Part model, mm, in its own coordinate system. A direction names the side the tool comes from. Round coordinates to 2 decimals unless told otherwise and drop trailing zeros. Order: outer loops, then holes, each group sorted by start corner. A loop starts at its lowest first (then second) coordinate and runs counter-clockwise, first axis right, second up. Notation, with made-up numbers: (66, -35) - (85, -35) arc R23 cw to (85, 0) - close; hole circle Ø11 at (74, 84.25). An arc over 180 degrees is marked (long way). Return JSON: item names as keys, results as strings. Group by question number.
Item 1: Tool access for faces 4 (the face through (-9.76, 2.57, 2.17)), 5 (the face through (0, 25, 0)): list every direction of +Z, -Z, +X, -X, +Y, -Y with a clear straight run to the whole face (end or side of a thin tool).
Item 2: Probe probe 1 along X at (y, z) = (13.5, 0); probe 2 along X at (y, z) = (3.15, 0); probe 3 along Y at (x, z) = (2, 1). List the from-to ranges inside material, lowest first.
Item 3: Saw through at B-B on y = 6.25. List the corners of the cut face in (x, z).
Item 4: Saw through at A-A on y = 2. List the corners of the cut face in (x, z).
Item 5: Drop flat-ended pins along their axis: pin 1 (12 mm diameter, centred on x = -1, z = -1.5, fed in from -Y); pin 2 (2 mm diameter, centred on y = 7.5, z = -9.5, fed in from +X); pin 3 (10 mm diameter, centred on y = 21, z = 10, fed in from -X). Give the stop position or say it passes through.
Item 6: Two-plate mould, pull along X, no slides. Class faces 1 (the face through (3.755, 11.933, 11.923)), 2 (the face through (0.9, 12.5, -2.86)), 3 (the face through (7.35, 0, -7.35)): released by +X, released by -X, zero draft, split by the parting line, or undercut.
```python
from build123d import *

# Parameters (mm, degrees)
SKETCH_1_R          = 12.5
EXTRUDE_1_DEPTH     = 25
SKETCH_2_R          = 10
CUT_EXTRUDE_1_DEPTH = 5
SKETCH_3_R          = 3
CUT_EXTRUDE_2_DEPTH = 15
CHAMFER_1_SIZE      = 0.2
FILLET_1_SIZE       = 1


with BuildPart() as part:
    # 草图1 → 凸台-拉伸1 (new body)
    with BuildSketch(Plane(origin=(0, 0, 0), x_dir=(1, 0, 0), z_dir=(0, 1, 0))):
        with Locations(Location((0, 0, 0), (0, 0, 270))):
            Circle(SKETCH_1_R)
    extrude(amount=EXTRUDE_1_DEPTH)

    # 草图2 → 切除-拉伸1 (cut)
    with BuildSketch(Plane.XZ):
        with Locations(Location((0, 0, 0), (0, 0, 270))):
            Circle(SKETCH_2_R)
    extrude(amount=-CUT_EXTRUDE_1_DEPTH, mode=Mode.SUBTRACT)

    # 草图3 → 切除-拉伸2 (cut)
    with BuildSketch(Plane.XZ.offset(-5)):
        with Locations(Location((0, 0, 0), (0, 0, 270))):
            Circle(SKETCH_3_R)
    extrude(amount=-CUT_EXTRUDE_2_DEPTH, mode=Mode.SUBTRACT)

    # 倒角1
    chamfer_1_edges = [part.edges().sort_by_distance(p)[0] for p in [
        (0, 5, 3),
        (0, 0, -12.5),
        (0, 0, 10),
    ]]
    chamfer(chamfer_1_edges, length=CHAMFER_1_SIZE)

    # 圆角1
    # a fillet whose section is not a circle: 1 mm, written as the material it takes off along each edge
    with BuildSketch(Plane(origin=(0, 25, 0), x_dir=(0, 0, 1), z_dir=(-1, 0, 0))) as fillet_1_piece_1:
        with BuildLine():
            Bezier((12.5, -FILLET_1_SIZE), (12.5, 0), (12.5 - FILLET_1_SIZE, 0), weights=[1, 0.818181818, 1])
            Line((12.5 - FILLET_1_SIZE, 0), (12.5, 0))
            Line((12.5, 0), (12.5, -FILLET_1_SIZE))
        make_face()
    revolve(axis=Axis((0, 25, 0), (0, 1, 0)), mode=Mode.SUBTRACT)


solid = part.part
```
Filled in:
{
 "1": {"face 4": "-Y", "face 5": "+Z, -Z, +X, -X, +Y"},
 "2": {"probe 1": "x = -12.5 to -3, 3 to 12.5", "probe 2": "x = -12.5 to -10, 10 to 12.5", "probe 3": "y = 20 to 25"},
 "3": {"outline": "circle Ø25 at (0, 0); hole circle Ø6 at (0, 0)"},
 "4": {"outline": "circle Ø25 at (0, 0); hole circle Ø20 at (0, 0)"},
 "5": {"pin 1": "stops at y = 5", "pin 2": "stops at x = 9.17", "pin 3": "stops at x = -11.46"},
 "6": {"face 1": "split by the parting line", "face 2": "undercut", "face 3": "zero draft"}
}
